Work out the finished part from the listing and answer in its coordinate system (mm). Round coordinates to 2 decimals unless told otherwise and drop trailing zeros. Loops run counter-clockwise (first coordinate to the right, second up) from the corner with the lowest first, then second, coordinate; pieces in that order, holes last. Notation, with made-up numbers: (-33, 5.25) - (18, 5.25) arc R18 ccw to (18, 22.25) - close; hole circle Ø2 at (78, -31). An arc over 180 degrees is marked (long way). Return JSON: item names as keys, results as strings.
from build123d import *

# Parameters (mm, degrees)
BOSS_EXTRUDE1_DEPTH           = 34.4
SKETCH2_W                     = 50
SKETCH2_H                     = 11.3
BOSS_EXTRUDE2_DEPTH           = 14
BOSS_EXTRUDE2_DRAFT           = 1
BOSS_EXTRUDE2_PROFILE_2_DEPTH = 14
BOSS_EXTRUDE2_PROFILE_2_DRAFT = 1
FILLET1_R                     = 5


with BuildPart() as part:
    # Sketch1 → Boss-Extrude1 (new body)
    with BuildSketch(Plane.XY):
        Polygon((45, 0), (50, 0), (50, 40), (0, 40), (0, 0), (5, 0), (5, 25), (45, 25), align=None)
    extrude(amount=BOSS_EXTRUDE1_DEPTH)


with BuildPart() as boss_extrude2_tool:
    # Sketch2 → Boss-Extrude2 (with draft: the straight prism first)
    with BuildSketch(Plane(origin=(0, 40, 0), x_dir=(1, 0, 0), z_dir=(0, 1, 0))):
        with Locations((25, -5.65)):
            Rectangle(SKETCH2_W, SKETCH2_H)
    extrude(amount=BOSS_EXTRUDE2_DEPTH)
    # Boss-Extrude2: the draft: its side faces are tilted about the plane it starts from
    boss_extrude2_sides = [boss_extrude2_tool.faces().sort_by_distance(p)[0] for p in [
        (0, 47, 5.65),
        (25, 47, 11.3),
        (50, 47, 5.65),
        (25, 47, 0),
    ]]
    draft(boss_extrude2_sides, Plane(origin=(0, 40, 0), x_dir=(1, 0, 0), z_dir=(0, 1, 0)), BOSS_EXTRUDE2_DRAFT)


with BuildPart() as part_1:
    add(part.part)

    # Boss-Extrude2: add boss_extrude2_tool
    add(boss_extrude2_tool.part)


with BuildPart() as boss_extrude2_profile_2_tool:
    # Sketch2 → Boss-Extrude2 profile 2 (with draft: the straight prism first)
    with BuildSketch(Plane(origin=(0, 40, 0), x_dir=(1, 0, 0), z_dir=(0, 1, 0))):
        with Locations((25, -28.75)):
            Rectangle(SKETCH2_W, SKETCH2_H)
    extrude(amount=BOSS_EXTRUDE2_PROFILE_2_DEPTH)
    # Boss-Extrude2 profile 2: the draft: its side faces are tilted about the plane it starts from
    boss_extrude2_profile_2_sides = [boss_extrude2_profile_2_tool.faces().sort_by_distance(p)[0] for p in [
        (25, 47, 34.4),
        (50, 47, 28.75),
        (25, 47, 23.1),
        (0, 47, 28.75),
    ]]
    draft(boss_extrude2_profile_2_sides, Plane(origin=(0, 40, 0), x_dir=(1, 0, 0), z_dir=(0, 1, 0)), BOSS_EXTRUDE2_PROFILE_2_DRAFT)


with BuildPart() as part_2:
    add(part_1.part)

    # Boss-Extrude2 profile 2: add boss_extrude2_profile_2_tool
    add(boss_extrude2_profile_2_tool.part)

    # Fillet1
    # the kernel refuses this fillet: 5 mm, written as the material it takes off along each edge
    with BuildSketch(Plane(origin=(50, -30, 34.4), x_dir=(-1, 0, 0), z_dir=(0, 1, 0)), Plane(origin=(0, 70, 0), x_dir=(0, 0, 1), z_dir=(0, -1, 0))) as fillet1_piece_1:
        with BuildLine():
            CenterArc((FILLET1_R, -FILLET1_R), FILLET1_R, 90, 90)
            Line((0, -FILLET1_R), (-FILLET1_R * 0.02, -FILLET1_R))
            Line((-FILLET1_R * 0.02, -FILLET1_R), (-FILLET1_R * 0.02, FILLET1_R * 0.02))
            Line((-FILLET1_R * 0.02, FILLET1_R * 0.02), (FILLET1_R, FILLET1_R * 0.02))
            Line((FILLET1_R, FILLET1_R * 0.02), (FILLET1_R, 0))
        make_face()
    extrude(amount=100, mode=Mode.SUBTRACT)
    with BuildSketch(Plane(origin=(50, -30, 0), x_dir=(-1, 0, 0), z_dir=(0, 1, 0)), Plane(origin=(0, 70, 34.4), x_dir=(0, 0, -1), z_dir=(0, -1, 0))) as fillet1_piece_2:
        with BuildLine():
            CenterArc((FILLET1_R, FILLET1_R), FILLET1_R, 180, 90)
            Line((0, FILLET1_R), (-FILLET1_R * 0.02, FILLET1_R))
            Line((-FILLET1_R * 0.02, FILLET1_R), (-FILLET1_R * 0.02, -FILLET1_R * 0.02))
            Line((-FILLET1_R * 0.02, -FILLET1_R * 0.02), (FILLET1_R, -FILLET1_R * 0.02))
            Line((FILLET1_R, -FILLET1_R * 0.02), (FILLET1_R, 0))
        make_face()
    extrude(amount=100, mode=Mode.SUBTRACT)


solid = part_2.part
1) Determine the mould class of faces 1 (the flat face through (25, 25, 17)), 2 (the flat face through (5, 12, 17)), 3 (the flat face through (47, 0, 17)), 4 (the cylindrical face through (1.5, 27.38, 32.97)) for opening direction X: pulls with the +X half, pulls with the -X half, needs draft (parallel to the pull), parting line crosses it, or undercut.
Verdict:
{"face 1": "undercut", "face 2": "undercut", "face 3": "needs draft", "face 4": "pulls with the -X half"}
2) Section A-A (y = 44) is taken. Give the vertices of the cut face in (x, z), and give its area (3 significant figures).
Verdict:
{"outline": "(0.07, 4.17) arc R5 ccw to (4.17, 0.07) - (45.83, 0.07) arc R5 ccw to (49.93, 4.17) - (49.93, 11.23) - (0.07, 11.23) - close; (0.07, 23.17) - (49.93, 23.17) - (49.93, 30.23) arc R5 ccw to (45.83, 34.33) - (4.17, 34.33) arc R5 ccw to (0.07, 30.23) - close", "area": "1,090 mm2"}
3) Section B-B (x = 33) is taken. Give the vertices of the cut face in (y, z).
Verdict:
{"outline": "(25, 0) - (40, 0) - (54, 0.24) - (54, 11.06) - (40, 11.3) - (40, 23.1) - (54, 23.34) - (54, 34.16) - (40, 34.4) - (25, 34.4) - close"}
4) Section C-C (z = 14) is taken. Give the vertices of the cut face in (x, y), and give its area (3 significant figures).
Verdict:
{"outline": "(0, 0) - (5, 0) - (5, 25) - (45, 25) - (45, 0) - (50, 0) - (50, 40) - (0, 40) - close", "area": "1,000 mm2"}
5) Flat-ended cylindrical pins translate along their axes: pin 1 (4 mm diameter, centred on x = 13, z = 25.5, fed in from -Y); pin 2 (2 mm diameter, centred on x = 32, y = 23, fed in from -Z); pin 3 (8 mm diameter, centred on x = 30.5, y = 47, fed in from +Z); pin 4 (3.5 mm diameter, centred on x = 14, z = 18.5, fed in from +Y). Find the tip coordinate at first contact, or state that the pin passes through.
Verdict:
{"pin 1": "stops at y = 25", "pin 2": "passes through", "pin 3": "stops at z = 34.35", "pin 4": "stops at y = 40"}
6) Section D-D (y = 13) is taken. Give the vertices of the cut face in (x, z).
Verdict:
{"outline": "(0, 5) arc R5 ccw to (5, 0) - (5, 34.4) arc R5 ccw to (0, 29.4) - close; (45, 0) arc R5 ccw to (50, 5) - (50, 29.4) arc R5 ccw to (45, 34.4) - close"}
7) Find the intervals of material crossed by L1, parallel to X at y = 24.5, z = 27; L2, parallel to Y at x = 27.5, z = 4; L3, parallel to Y at x = 9.5, z = 22.5, in increasing order.
Verdict:
{"L1": "x = 0 to 5, 45 to 50", "L2": "y = 25 to 54", "L3": "y = 25 to 40"}
